Geometry check sheet. Reference: drawing and pictorial views, mm from the part's lowest x, y, z. Give positions to 0.01 mm unless a question says otherwise; leave off trailing zeros. Loops run counter-clockwise (first coordinate to the right, second up) from the corner with the lowest first, then second, coordinate; pieces in that order, holes last. Notation, with made-up numbers: M 50.5,15 L 57.5,15 A13 ccw 57.5,35 Z; hole C 57,31 d8. An arc over 180 degrees is marked long. Use CSV: the item, a comma, the result in double quotes.
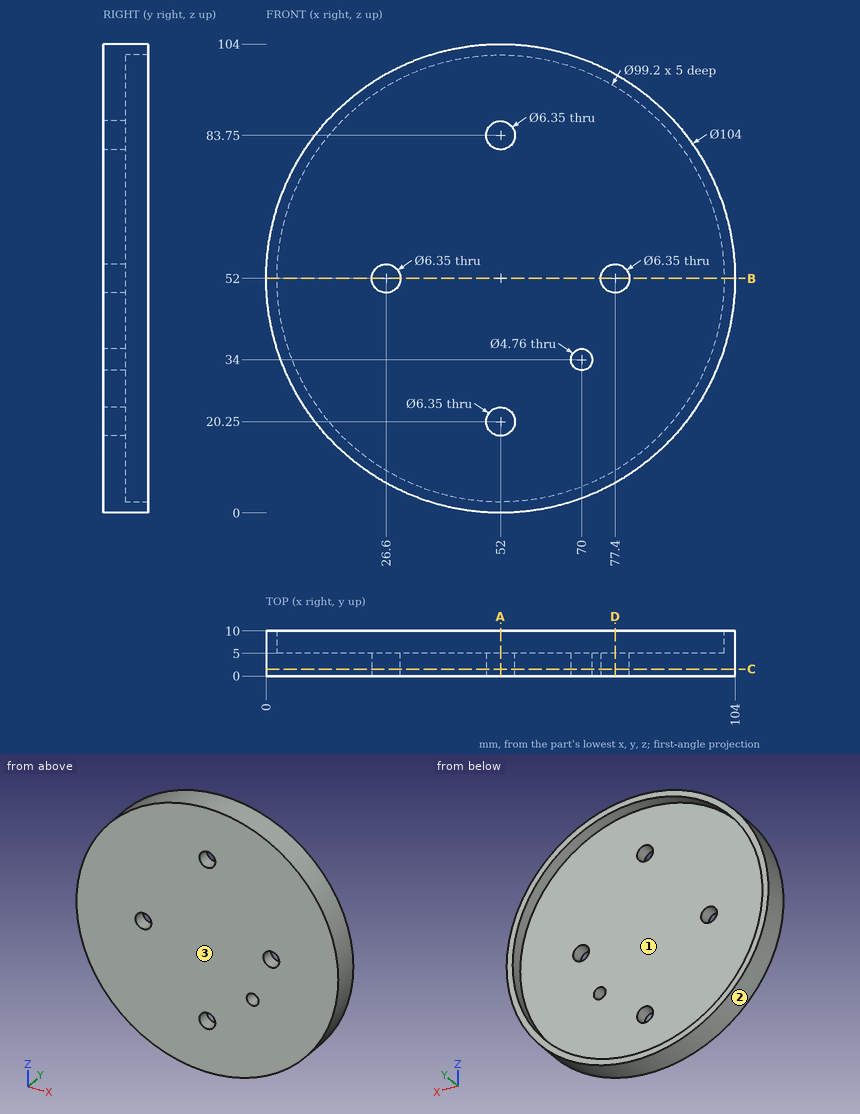
(1) Depth check by flat-ended pin: pin 1 Ø6 at (x, y) = (22, 2) entering from +Z; pin 2 Ø1.5 at (y, z) = (3.5, 40) entering from -X; pin 3 Ø5 at (x, y) = (39.5, 2) entering from -Z; pin 4 Ø7.5 at (x, z) = (26.6, 52) entering from -Y. Enter the tip coordinate at first touch or a pass-through.
Calculated:
pin 1,"stops at z = 96.44"
pin 2,"stops at x = 1.23"
pin 3,"stops at z = 0.97"
pin 4,"stops at y = 0"
(2) Section check D-D on x = 77.4. Record the cut outline in (y, z) (3 decimals), plus the area to 3 significant figures.
Calculated:
outline,"M 0,6.626 L 10,6.626 L 10,9.397 L 5,9.397 L 5,48.825 L 0,48.825 Z; M 0,55.175 L 5,55.175 L 5,94.603 L 10,94.603 L 10,97.374 L 0,97.374 Z"
area,"450 mm²"
(3) Section check B-B on z = 52. Record the cut outline in (x, y) (3 decimals), plus the area to 4 significant figures.
Calculated:
outline,"M 0,0 L 23.425,0 L 23.425,5 L 2.4,5 L 2.4,10 L 0,10 Z; M 29.775,0 L 74.225,0 L 74.225,5 L 29.775,5 Z; M 80.575,0 L 104,0 L 104,10 L 101.6,10 L 101.6,5 L 80.575,5 Z"
area,"480.5 mm²"
(4) Section check C-C on y = 1.5. Record the cut outline in (x, z) (3 decimals).
Calculated:
outline,"C 52,52 d104; hole C 26.6,52 d6.35; hole C 52,20.25 d6.35; hole C 52,83.75 d6.35; hole C 70,34 d4.76; hole C 77.4,52 d6.35"
(5) Scan lines: L1, parallel to X at y = 1.7, z = 52 (3 decimals); L2, parallel to X at y = 7.3, z = 52. Record each from-to range of solid material in increasing order. Write a range as from..to.
Calculated:
L1,"x = 0..23.425, 29.775..74.225, 80.575..104"
L2,"x = 0..2.4, 101.6..104"
(6) Section check A-A on x = 52. Record the cut outline in (y, z) (3 decimals).
Calculated:
outline,"M 0,0 L 10,0 L 10,2.4 L 5,2.4 L 5,17.075 L 0,17.075 Z; M 0,23.425 L 5,23.425 L 5,80.575 L 0,80.575 Z; M 0,86.925 L 5,86.925 L 5,101.6 L 10,101.6 L 10,104 L 0,104 Z"
(7) Mould release check, pull along Z, two halves, no side actions. Record for the marked faces 1, 2 and 3: released by +Z, released by -Z, zero draft, split by the parting line, or undercut.
Calculated:
face 1,"undercut"
face 2,"split by the parting line"
face 3,"zero draft"
